```python
from build123d import *

# Parameters (mm, degrees)
F1_DEPTH = 10
F3_DEPTH = 20
F5_DEPTH = 7.5358984849


with BuildPart() as f1:
    # F0 (on Right) → F1 (new body, symmetric)
    with BuildSketch(Plane.YZ):
        with BuildLine():
            ThreePointArc((-20.8296291314, -1.2940952255), (-20.9926964007, 0.2701530127), (-20.6617935804, 1.8076727064))
            ThreePointArc((-20.6617935804, 1.8076727064), (-20.6809628133, 3.646611731), (-20.0339954379, 5.3680928987))
            ThreePointArc((-20.0339954379, 5.3680928987), (-19.7335450365, 7.1824230098), (-18.7974744816, 8.7654063047))
            ThreePointArc((-18.7974744816, 8.7654063047), (-11.7433151518, 12.5315389352), (-10.0940139115, 4.7069159885))
            ThreePointArc((-10.0940139115, 4.7069159885), (-10.3366188286, 3.7622215766), (-10.7580105429, 2.8826002371))
            ThreePointArc((-10.7580105429, 2.8826002371), (-10.8328852831, 1.9101299543), (-11.0951304678, 0.9706981363))
            ThreePointArc((-11.0951304678, 0.9706981363), (-11.0027569299, -0.1660171642), (-11.1703708686, -1.2940952255))
            ThreePointArc((-11.1703708686, -1.2940952255), (-8, -5.4258029827), (-4.8296291314, -1.2940952255))
            ThreePointArc((-4.8296291314, -1.2940952255), (0, 5), (4.8296291314, -1.2940952255))
            ThreePointArc((4.8296291314, -1.2940952255), (5.8902893032, -3.1312125326), (7.7274066103, -2.0705523608))
            ThreePointArc((7.7274066103, -2.0705523608), (7.8547454968, 1.517555001), (6.4, 4.8))
            ThreePointArc((6.4, 4.8), (6.211145618, 6.894427191), (8, 8))
            Line((8, 8), (18, 8))
            ThreePointArc((18, 8), (19.4142135624, 8.5857864376), (20, 10))
            Line((20, 10), (20, 16))
            Line((20, 16), (14, 16))
            ThreePointArc((14, 16), (12.8284271247, 13.1715728753), (10, 12))
            Line((10, 12), (-6, 12))
            Line((-6, 12), (-6, 14))
            ThreePointArc((-6, 14), (-8.4616553345, 13.9180532248), (-10.8315712253, 14.5888444966))
            ThreePointArc((-10.8315712253, 14.5888444966), (-16.0570828985, 14.9079319058), (-20.135090638, 11.625))
            ThreePointArc((-20.135090638, 11.625), (-22.5254325043, 5.7591136901), (-23.2438614431, -0.5342332969))
            ThreePointArc((-23.2438614431, -0.5342332969), (-22.7288527683, -3.1131272319), (-20.8296291314, -1.2940952255))
        make_face()
    extrude(amount=F1_DEPTH, both=True)

    # F2 (on face) → F3 (cut, through all)
    with BuildSketch(Plane.YZ.offset(10)):
        with BuildLine():
            Line((1, 10), (-3, 10))
            ThreePointArc((-3, 10), (-4, 9), (-3, 8))
            Line((-3, 8), (1, 8))
            ThreePointArc((1, 8), (2, 9), (1, 10))
        make_face()
    extrude(amount=-F3_DEPTH, mode=Mode.SUBTRACT)

    # F4 (on face) → F5 (cut, up to face)
    with BuildSketch(Plane(origin=(0, 20, 0), x_dir=(-1, 0, 0), z_dir=(0, 1, 0))):
        with BuildLine():
            Line((6.3245553203, 16), (-6.3245553203, 16))
            ThreePointArc((-6.3245553203, 16), (0, 14), (6.3245553203, 16))
        make_face()
    extrude(amount=-F5_DEPTH, mode=Mode.SUBTRACT)


solid = f1.part
```
Design review of the part built by this model. Coordinates are the model's own, in mm. A direction names the side the tool comes from. Coordinates: 2 decimals unless noted, no trailing zeros. Loops run counter-clockwise (first coordinate to the right, second up) from the corner with the lowest first, then second, coordinate; pieces in that order, holes last. Notation, with made-up numbers: (77, -16.5) - (105, -16.5) arc R16 cw to (105, 6.5) - close; hole circle Ø2 at (16.25, 21). An arc over 180 degrees is marked (long way). Use CSV: the item, a comma, the result in double quotes. Start each with the question number.
1) Consider section D-D on y = 14.5. Write out the cut boundary in (x, z), then the cut area to 3 significant figures.
2) Consider section A-A on z = 0. Write out the cut boundary in (x, y), then the cut area to 3 significant figures.
3) Consider section C-C on x = 7.25. Write out the cut boundary in (y, z) (3 decimals).
4) The part is to be moulded in two halves that separate along Z. For faces 1 (the cylindrical face through (0.14, 7.864, 1.468)), 2 (the flat face through (0, 20, 12)), 3 (the cylindrical face through (0.14, 19.4, 8.57)), 4 (the flat face through (0, -1, 8)), say which applies: +Z half, -Z half, draft (parallel to the pull), parting line (faces both ways), or undercut.
5) Consider section B-B on y = 0. Write out the cut boundary in (x, z), then the cut area to 3 significant figures.
6) Tool access review of faces 5 (the flat face through (0, -6, 13)), 6 (the flat face through (0, 13, 8)), 7 (the flat face through (10, -2, 7.7)), 8 (the cylindrical face through (0.14, -10.33, 3.78)): name each direction out of +Z, -Z, +X, -X, +Y, -Y from which nothing blocks a thin tool from reaching the whole face with its end or side.
7) Wall thickness on L1, parallel to Y at x = -2, z = 0; L2, parallel to Z at x = 0.5, y = 0; L3, parallel to Y at x = -0.25, z = 3.5: over which ranges is each line inside the solid? List them lowest first. Write a range as from..to.
8) For pin 1 Ø3 at (x, y) = (5, 13) entering from -Z; pin 2 Ø10 at (x, y) = (1.5, 1.5) entering from +Z; pin 3 Ø8 at (x, z) = (2, 10) entering from -Y, all flat-tipped, find the tip position at first contact; note any pin that passes through.
Geometry says:
1,outline,"(-10, 8) - (10, 8) - (10, 16) - (6.32, 16) arc R11 cw to (-6.32, 16) - (-10, 16) - close"
1,area,"143 mm^2"
2,outline,"(-10, -23.25) - (10, -23.25) - (10, -21) - (-10, -21) - close; (-10, -11) - (10, -11) - (10, -5) - (-10, -5) - close; (-10, 5) - (10, 5) - (10, 8) - (-10, 8) - close"
2,area,"225 mm^2"
3,outline,"(-23.244, -0.534) arc R1.5 ccw (long way) to (-20.83, -1.294) arc R5 cw to (-20.662, 1.808) arc R5 cw to (-20.034, 5.368) arc R5 cw to (-18.797, 8.765) arc R5 cw (long way) to (-10.094, 4.707) arc R5 cw to (-10.758, 2.883) arc R5 cw to (-11.095, 0.971) arc R5 cw to (-11.17, -1.294) arc R3.282 ccw (long way) to (-4.83, -1.294) arc R5 cw (long way) to (4.83, -1.294) arc R1.5 ccw to (7.727, -2.071) arc R8 ccw to (6.4, 4.8) arc R2 cw to (8, 8) - (18, 8) arc R2 ccw to (20, 10) - (20, 16) - (14, 16) arc R4 cw to (10, 12) - (-6, 12) - (-6, 14) arc R8 cw to (-10.832, 14.589) arc R7.25 ccw to (-20.135, 11.625) arc R23.25 ccw to start; hole (-3, 8) - (1, 8) arc R1 ccw to (1, 10) - (-3, 10) arc R1 ccw to start"
4,face 1,"undercut"
4,face 2,"draft"
4,face 3,"-Z half"
4,face 4,"undercut"
5,outline,"(-10, 5) - (10, 5) - (10, 8) - (-10, 8) - close; (-10, 10) - (10, 10) - (10, 12) - (-10, 12) - close"
5,area,"100 mm^2"
6,face 5,"+Z, +X, -X"
6,face 6,"-Z, +X, -X, +Y"
6,face 7,"+Z, -Z, +X, +Y, -Y"
6,face 8,"+X, -X"
7,L1,"-23.25..-21, -11..-5, 5..8"
7,L2,"5..8, 10..12"
7,L3,"-22.99..-20.7, -10.44..-3.57, 3.57..7.19"
8,pin 1,"z = 8"
8,pin 2,"z = 12"
8,pin 3,"y = -22.46"
